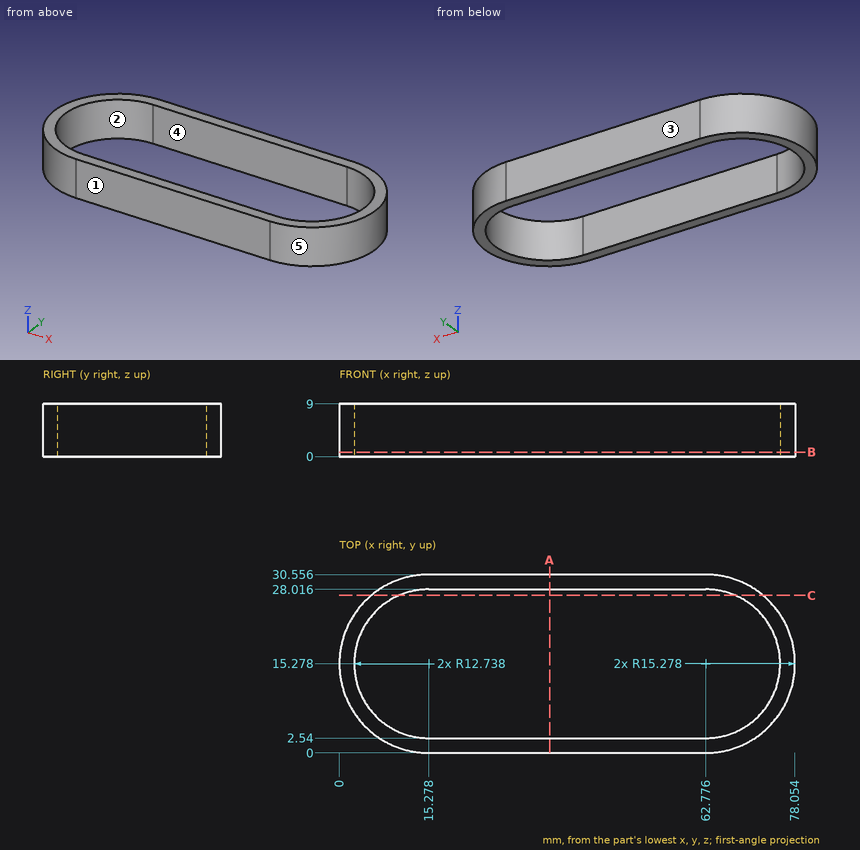
Answer from the drawing. Dimensions are ordinates in mm from the lowest x, y and z of the part. A direction names the side the tool comes from. Give positions to 0.01 mm unless a question says otherwise; leave off trailing zeros. Loops run counter-clockwise (first coordinate to the right, second up) from the corner with the lowest first, then second, coordinate; pieces in that order, holes last. Notation, with made-up numbers: (70, -31.5) -> (101, -31.5) arc R34 ccw to (101, -1.5) -> close; hole circle Ø7 at (33.25, 50.25). An arc over 180 degrees is marked (long way). Answer as CSV lines item,"result".
Item 1: Find section A-A on x = 36. Give the vertices of the cut face in (y, z), plus the area to 3 significant figures.
Returned:
outline,"(0, 0) -> (2.54, 0) -> (2.54, 9) -> (0, 9) -> close; (28.02, 0) -> (30.56, 0) -> (30.56, 9) -> (28.02, 9) -> close"
area,"45.7 mm²"
Item 2: Find section B-B on z = 0.75. Give the vertices of the cut face in (x, y), plus the area to 3 significant figures.
Returned:
outline,"(15.28, 0) -> (62.78, 0) arc R15.28 ccw to (62.78, 30.56) -> (15.28, 30.56) arc R15.28 ccw to start; hole (15.28, 2.54) -> (62.78, 2.54) arc R12.74 ccw to (62.78, 28.02) -> (15.28, 28.02) arc R12.74 ccw to start"
area,"465 mm²"
Item 3: Determine the mould class of the marked faces 3, 4 and 5 for opening direction X: +X half, -X half, draft (parallel to the pull), parting line (faces both ways), or undercut.
Returned:
face 3,"draft"
face 4,"undercut"
face 5,"+X half"
Item 4: Consider line 1 (Y direction, x = 27, z = 1.75); line 2 (X direction, y = 15.5, z = 2.5); line 3 (Y direction, x = 66, z = 3.5) (1 decimal). Determine where each line is inside the solid, lowest interval first. Write a range as [from, to].
Returned:
line 1,"y = [0, 2.54], [28.02, 30.56]"
line 2,"x = [0, 2.54], [75.51, 78.05]"
line 3,"y = [0.3, 3], [27.6, 30.2]"
Item 5: Each of these flat-tipped pins is pushed along its axis until it touches: pin 1 (3 mm diameter, centred on y = 25, z = 3.5, fed in from -X); pin 2 (10 mm diameter, centred on x = 56, y = 21.5, fed in from +Z); pin 3 (5 mm diameter, centred on y = 8, z = 6, fed in from -X). Where does it stop, or does it pass through?
Returned:
pin 1,"stops at x = 2.4"
pin 2,"passes through"
pin 3,"stops at x = 0.77"
Item 6: For the marked faces 1 and 2, determine the directions among +Z, -Z, +X, -X, +Y, -Y from which every point of the face is accessible in a straight line to the end or side of a thin tool.
Returned:
face 1,"+Z, -Z, +X, -X, -Y"
face 2,"+Z, -Z"
Item 7: Find section C-C on y = 27. Give the vertices of the cut face in (x, z) (1 decimal).
Returned:
outline,"(5.5, 0) -> (10.3, 0) -> (10.3, 9) -> (5.5, 9) -> close; (67.8, 0) -> (72.6, 0) -> (72.6, 9) -> (67.8, 9) -> close"
